The listing builds one solid part. Answer for the finished solid, in the listing's coordinates (mm). A direction names the side the tool comes from. Coordinates: 2 decimals unless noted, no trailing zeros. Write each loop counter-clockwise with the first axis right and the second up, starting at its lowest first coordinate (ties: lowest second). Pieces come first, ordered by that corner, then holes.
(1) The part is cut by section D-D on x = 6.35. Determine the outline of the cut face in (y, z), plus the area to 3 significant figures.
(2) The part is cut by section B-B on y = 2. Determine the outline of the cut face in (x, z).
(3) For a pull along X with two mould halves and no side action, classify faces 1 (the cylindrical face through (96.936, -11.448, 24.325)), 2 (the flat face through (6, 0, 19.05)) as +X half, -X half, draft (parallel to the pull), parting line (faces both ways), or undercut.
(4) The part is cut by section A-A on y = 14.5. Determine the outline of the cut face in (x, z), plus the area to 3 significant figures.
(5) Given P1, Ø6.5, axis at x = 51.48, z = 29.52, coming from the -Y side; P2, Ø6.5, axis at x = 96.5, z = 26.5, coming from the +Y side; P3, Ø15.5, axis at y = 4, z = 1.5, coming from the -X side; P4, Ø6.5, axis at x = 95.25, z = 25.4, coming from the +Y side, each flat-ended and moving along its own axis, determine where each tip first touches the part or whether it passes through.
(6) The part is cut by section C-C on z = -25.4. Determine the outline of the cut face in (x, y).
(7) Which of the six approach directions +Z, -Z, +X, -X, +Y, -Y give full straight-line access (tool end or side, diameter ignored) to faces 3 (the cylindrical face through (50.089, 21.593, -0.59)), 4 (the cylindrical face through (3.916, 10.292, 28.574)), 5 (the flat face through (6, -12.7, 29)), 6 (the flat face through (6, 0, -19.05)), 7 (the flat face through (88.9, 13, -1))?
(8) Straight lines are drawn through the part: line 1 (Z direction, x = 6, y = 14); line 2 (X direction, y = -11.15, z = 25.4); line 3 (X direction, y = 2, z = 31.5). For each, find the intervals that lie inside material, in ascending order.
from build123d import *

# Parameters (mm, degrees)
BOSS_EXTRUDE1_DEPTH     = 101.6
SKETCH2_R               = 2
CUT_EXTRUDE1_DEPTH      = 120.381228758
SKETCH3_W               = 76.2
SKETCH3_H               = 62.425931944
CUT_EXTRUDE2_DEPTH      = 133.301446423
BOSS_EXTRUDE2_START     = -76.2
BOSS_EXTRUDE2_DEPTH     = 76.2
CUT_EXTRUDE3_DEPTH      = 27.94
CUT_EXTRUDE3_DEPTH_BACK = 19.05
SKETCH5_R               = 4
SKETCH6_W               = 38.1
SKETCH6_H               = 50.8
CUT_EXTRUDE4_DEPTH      = 115.668403311
SKETCH9_R               = 5
CUT_EXTRUDE6_DEPTH      = 15.24
SKETCH10_R              = 2.5
CUT_EXTRUDE7_DEPTH      = 113.708475404


with BuildPart() as part:
    # Sketch1 → Boss-Extrude1 (new body)
    with BuildSketch(Plane(origin=(0, 0, 0), x_dir=(0, 0, -1), z_dir=(1, 0, 0))):
        with BuildLine():
            Line((-38.1, 37.076578626), (-38.1, -12.7))
            Line((-38.1, -12.7), (38.1, -12.7))
            Line((38.1, -12.7), (38.1, 37.076578626))
            ThreePointArc((38.1, 37.076578626), (0, 21.59), (-38.1, 37.076578626))
        make_face()
    extrude(amount=BOSS_EXTRUDE1_DEPTH)

    # Sketch2 → Cut-Extrude1 (cut, through all)
    with BuildSketch(Plane(origin=(0, -12.7, 0), x_dir=(-1, 0, 0), z_dir=(0, -1, 0))):
        with Locations(Location((-6.35, -25.4, 0), (0, 0, 90))):
            Circle(SKETCH2_R)
        with Locations(Location((-6.35, 25.4, 0), (0, 0, 90))):
            Circle(SKETCH2_R)
        with Locations(Location((-95.25, -25.4, 0), (0, 0, 90))):
            Circle(SKETCH2_R)
        with Locations(Location((-95.25, 25.4, 0), (0, 0, 90))):
            Circle(SKETCH2_R)
    extrude(amount=-CUT_EXTRUDE1_DEPTH, mode=Mode.SUBTRACT)

    # Sketch3 → Cut-Extrude2 (cut, through all)
    with BuildSketch(Plane(origin=(0, 0, -38.1), x_dir=(-1, 0, 0), z_dir=(0, 0, -1))):
        with Locations((-50.8, -12.7)):
            Rectangle(SKETCH3_W, SKETCH3_H)
    extrude(amount=-CUT_EXTRUDE2_DEPTH, mode=Mode.SUBTRACT)

    # Sketch4 → Boss-Extrude2 (add)
    with BuildSketch(Plane(origin=(101.6, 0, 0), x_dir=(0, 0, -1), z_dir=(1, 0, 0)).offset(BOSS_EXTRUDE2_START)):
        with BuildLine():
            Line((-38.1, 37.076578626), (-38.1, 33.602905029))
            ThreePointArc((-38.1, 33.602905029), (0, 19.05), (38.1, 33.602905029))
            Line((38.1, 33.602905029), (38.1, 37.076578626))
            ThreePointArc((38.1, 37.076578626), (0, 21.59), (-38.1, 37.076578626))
        make_face()
    extrude(amount=BOSS_EXTRUDE2_DEPTH)

    # Sketch5 → Cut-Extrude3 (cut, two sides: drawn at the far end of the back side and taken through both)
    with BuildSketch(Plane(origin=(0, 17.78, 0), x_dir=(-1, 0, 0), z_dir=(0, -1, 0)).offset(-CUT_EXTRUDE3_DEPTH_BACK)):
        with Locations(Location((-95.25, 25.4, 0), (0, 0, 90))):
            Circle(SKETCH5_R)
        with Locations(Location((-6.35, 25.4, 0), (0, 0, 90))):
            Circle(SKETCH5_R)
        with Locations(Location((-6.35, -25.4, 0), (0, 0, 90))):
            Circle(SKETCH5_R)
        with Locations(Location((-95.25, -25.4, 0), (0, 0, 90))):
            Circle(SKETCH5_R)
    extrude(amount=CUT_EXTRUDE3_DEPTH + CUT_EXTRUDE3_DEPTH_BACK, mode=Mode.SUBTRACT)

    # Sketch6 → Cut-Extrude4 (cut, through all)
    with BuildSketch(Plane(origin=(101.6, 0, 0), x_dir=(0, 0, -1), z_dir=(1, 0, 0))):
        with Locations((0, -12.7)):
            Rectangle(SKETCH6_W, SKETCH6_H)
    extrude(amount=-CUT_EXTRUDE4_DEPTH, mode=Mode.SUBTRACT)

    # Sketch9 → Cut-Extrude6 (cut)
    with BuildSketch(Plane(origin=(0, 38.1, 0), x_dir=(-1, 0, 0), z_dir=(0, -1, 0))):
        with Locations(Location((-51.475148777, -29.522267927, 0), (0, 0, 270))):
            Circle(SKETCH9_R)
    extrude(amount=CUT_EXTRUDE6_DEPTH, mode=Mode.SUBTRACT)

    # Sketch10 → Cut-Extrude7 (cut, through all)
    with BuildSketch(Plane(origin=(0, 17.78, 0), x_dir=(-1, 0, 0), z_dir=(0, -1, 0))):
        with Locations(Location((-51.475148777, -29.522267927, 0), (0, 0, 90))):
            Circle(SKETCH10_R)
    extrude(amount=-CUT_EXTRUDE7_DEPTH, mode=Mode.SUBTRACT)


solid = part.part
Model answer:
1. outline: (-12.7, -38.1) - (37.08, -38.1) arc R54.61 cw to (30.18, -29.4) - (-10.16, -29.4) - (-10.16, -27.4) - (-12.7, -27.4) - close; (-12.7, -23.4) - (-10.16, -23.4) - (-10.16, -21.4) - (25.96, -21.4) arc R54.61 cw to (25.96, 21.4) - (-10.16, 21.4) - (-10.16, 23.4) - (-12.7, 23.4) - (-12.7, 19.05) - (12.7, 19.05) - (12.7, -19.05) - (-12.7, -19.05) - close; (-12.7, 27.4) - (-10.16, 27.4) - (-10.16, 29.4) - (30.18, 29.4) arc R54.61 cw to (37.08, 38.1) - (-12.7, 38.1) - close
1. area: 1,380 mm2
2. outline: (0, -38.1) - (12.7, -38.1) - (12.7, -19.05) - (0, -19.05) - close; (0, 19.05) - (12.7, 19.05) - (12.7, 38.1) - (0, 38.1) - close; (88.9, -38.1) - (101.6, -38.1) - (101.6, -19.05) - (88.9, -19.05) - close; (88.9, 19.05) - (101.6, 19.05) - (101.6, 38.1) - (88.9, 38.1) - close; hole circle Ø8 at (6.35, -25.4); hole circle Ø8 at (6.35, 25.4); hole circle Ø8 at (95.25, -25.4); hole circle Ø8 at (95.25, 25.4)
3. face 1: undercut
3. face 2: draft
4. outline: (0, -38.1) - (12.7, -38.1) - (12.7, 38.1) - (0, 38.1) - close; (88.9, -38.1) - (101.6, -38.1) - (101.6, 38.1) - (88.9, 38.1) - close; hole circle Ø8 at (6.35, -25.4); hole circle Ø8 at (6.35, 25.4); hole circle Ø8 at (95.25, -25.4); hole circle Ø8 at (95.25, 25.4)
4. area: 1,730 mm2
5. P1: stops at y = 18.51
5. P2: stops at y = 30.4
5. P3: passes through
5. P4: stops at y = -10.16
6. outline: (0, -12.7) - (4.35, -12.7) - (4.35, -10.16) - (2.35, -10.16) - (2.35, 27.86) - (0, 27.86) - close; (8.35, -12.7) - (12.7, -12.7) - (12.7, 18.51) - (88.9, 18.51) - (88.9, -12.7) - (93.25, -12.7) - (93.25, -10.16) - (91.25, -10.16) - (91.25, 27.86) - (10.35, 27.86) - (10.35, -10.16) - (8.35, -10.16) - close; (97.25, -12.7) - (101.6, -12.7) - (101.6, 27.86) - (99.25, 27.86) - (99.25, -10.16) - (97.25, -10.16) - close
7. face 3: +X, -X, +Y
7. face 4: +Y
7. face 5: +Z, -Z, +X, -X, -Y
7. face 6: +X, -X, -Y
7. face 7: +Z, -Z, -Y
8. line 1: z = -38.1 to -29.38, -21.42 to 21.42, 29.38 to 38.1
8. line 2: x = 0 to 4.35, 8.35 to 12.7, 88.9 to 93.25, 97.25 to 101.6
8. line 3: x = 0 to 12.7, 88.9 to 101.6
